from build123d import *

# Parameters (mm, degrees)
SKETCH_2_R      = 1.6
SKETCH_2_W      = 5
SKETCH_2_H      = 2
SKETCH_2_W_2    = 25.8
SKETCH_2_H_2    = 5
EXTRUDE_1_DEPTH = 1.6
SKETCH_3_W      = 5
SKETCH_3_H      = 25
SKETCH_3_W_2    = 7.5
SKETCH_3_H_2    = 5
SKETCH_3_W_3    = 8
SKETCH_3_H_3    = 4.5
SKETCH_3_W_4    = 25
SKETCH_3_H_4    = 24.5
EXTRUDE_2_DEPTH = 2
SKETCH_4_R      = 1.5
EXTRUDE_3_DEPTH = 5
SKETCH_5_W      = 5.2
SKETCH_5_H      = 3
SKETCH_5_W_2    = 4.3
SKETCH_5_H_2    = 4.3
SKETCH_5_W_3    = 3
SKETCH_5_H_3    = 5.2
EXTRUDE_4_DEPTH = 2


with BuildPart() as part:
    # 草图2 → 凸台-拉伸1 (new body)
    with BuildSketch(Plane(origin=(0, 0, 0), x_dir=(1, 0, 0), z_dir=(0, 1, 0))):
        Polygon((0, 0), (0, -53), (8, -53), (8, -37), (26, -37), (26, -53), (91, -53), (91, 0), align=None)
        with Locations(Location((3, -50, 0), (0, 0, 270))):
            Circle(SKETCH_2_R, mode=Mode.SUBTRACT)
        with Locations(Location((3, -3, 0), (0, 0, 270))):
            Circle(SKETCH_2_R, mode=Mode.SUBTRACT)
        with Locations(Location((88, -30, 0), (0, 0, 270))):
            Circle(SKETCH_2_R, mode=Mode.SUBTRACT)
        with Locations(Location((88, -50, 0), (0, 0, 270))):
            Circle(SKETCH_2_R, mode=Mode.SUBTRACT)
        with Locations((14, -33)):
            Rectangle(SKETCH_2_W, SKETCH_2_H, mode=Mode.SUBTRACT)
        with Locations((70.1, -38.9)):
            Rectangle(SKETCH_2_W_2, SKETCH_2_H_2, mode=Mode.SUBTRACT)
    extrude(amount=EXTRUDE_1_DEPTH)

    # 草图3 → 凸台-拉伸2 (add)
    with BuildSketch(Plane(origin=(0, 1.6, 0), x_dir=(1, 0, 0), z_dir=(0, 1, 0))):
        with Locations((2.5, -26.5)):
            Rectangle(SKETCH_3_W, SKETCH_3_H)
        with Locations((14.05, -18)):
            Rectangle(SKETCH_3_W_2, SKETCH_3_H_2)
        with Locations((22, -32.25)):
            Rectangle(SKETCH_3_W_3, SKETCH_3_H_3)
        with Locations((69.5, -18)):
            Rectangle(SKETCH_3_W_4, SKETCH_3_H_2)
        with Locations((88.5, -13.75)):
            Rectangle(SKETCH_3_W, SKETCH_3_H_4)
    extrude(amount=EXTRUDE_2_DEPTH)

    # 草图4 → 凸台-拉伸3 (add)
    with BuildSketch(Plane(origin=(0, 1.6, 0), x_dir=(1, 0, 0), z_dir=(0, 1, 0))):
        with Locations(Location((34.5, -38.8, 0), (0, 0, 270))):
            Circle(SKETCH_4_R)
        with Locations(Location((38.1, -38.8, 0), (0, 0, 270))):
            Circle(SKETCH_4_R)
        with Locations(Location((41.7, -38.8, 0), (0, 0, 270))):
            Circle(SKETCH_4_R)
    extrude(amount=EXTRUDE_3_DEPTH)

    # 草图5 → 凸台-拉伸4 (add)
    with BuildSketch(Plane(origin=(0, 1.6, 0), x_dir=(1, 0, 0), z_dir=(0, 1, 0))):
        with Locations((39.5, -43.5)):
            Rectangle(SKETCH_5_W, SKETCH_5_H)
        with Locations((49.05, -44.25)):
            Rectangle(SKETCH_5_W_2, SKETCH_5_H_2)
        with Locations((53.1, -40.8)):
            Rectangle(SKETCH_5_W_3, SKETCH_5_H_3)
    extrude(amount=EXTRUDE_4_DEPTH)


solid = part.part
Part model, mm, in its own coordinate system. A direction names the side the tool comes from. Coordinates: 2 decimals unless noted, no trailing zeros. Loops run counter-clockwise (first coordinate to the right, second up) from the corner with the lowest first, then second, coordinate; pieces in that order, holes last. Notation, with made-up numbers: M 16,75 L 75,75 A10 cw 75,91 Z; hole C 23.5,51.25 d4. An arc over 180 degrees is marked long. Use a Markdown table: item, result. Add a question column.
Q1. Pin check, flat tips, straight feed: P1, Ø10, axis at x = 81.5, z = 20, coming from the -Y side; P2, Ø1.5, axis at x = 52.5, z = 41, coming from the +Y side; P3, Ø1, axis at x = 60.5, y = 4, coming from the -Z side; P4, Ø0.8, axis at x = 14, y = 0.5, coming from the +Z side. Stop position of each tip, or through.
Q2. Cut at D-D (x = 38.1). Write the cut outline in (y, z), and give its area (3 significant figures).
Q3. Probe L1, parallel to X at y = 3, z = 17; L2, parallel to X at y = 1.1, z = 50; L3, parallel to Z at x = 62.5, y = 1.5. List the from-to ranges inside material, lowest first.
Q4. Which spindle directions (+Z, -Z, +X, -X, +Y, -Y) get a long thin tool onto all of the face, cutting with end or side? Do faces 1 (the flat face through (22, 3, 34.5)), 2 (the flat face through (5, 3, 27)), 3 (the flat face through (2, 3, 14)). Say none if no direction does.
Q5. Cut at C-C (y = 5.5). Write the cut outline in (x, z), and give its area (3 significant figures).
Q6. Mould opens along Z. For faces 4 (the flat face through (69, 3.6, 18)), 5 (the flat face through (49, 3, 42.1)), 6 (the cylindrical face through (88.481, 0.789, 51.526)) say: +Z half, -Z half, draft (parallel to the pull), parting line (faces both ways), or undercut.
Q7. Cut at B-B (z = 3). Write the cut outline in (x, y).
Q8. Cut at A-A (x = 69). Write the cut outline in (y, z).
Worked out:
| question | item | result |
|---|---|---|
| 1 | P1 | stops at y = 0 |
| 1 | P2 | stops at y = 3.6 |
| 1 | P3 | stops at z = 15.5 |
| 1 | P4 | stops at z = 37 |
| 2 | outline | M 0,0 L 1.6,0 L 1.6,37.3 L 6.6,37.3 L 6.6,40.3 L 1.6,40.3 L 1.6,42 L 3.6,42 L 3.6,45 L 1.6,45 L 1.6,53 L 0,53 Z |
| 2 | area | 106 mm2 |
| 3 | L1 | x = 0 to 5, 10.3 to 17.8, 57 to 82, 86 to 91 |
| 3 | L2 | x = 0 to 1.4, 4.6 to 8, 26 to 86.4, 89.6 to 91 |
| 3 | L3 | z = 0 to 36.4, 41.4 to 53 |
| 4 | face 1 | +Z, +X, +Y |
| 4 | face 2 | +Z, -Z, +Y |
| 4 | face 3 | -Z, -X, +Y |
| 5 | outline | C 34.5,38.8 d3; C 38.1,38.8 d3; C 41.7,38.8 d3 |
| 5 | area | 21.2 mm2 |
| 6 | face 4 | draft |
| 6 | face 5 | -Z half |
| 6 | face 6 | undercut |
| 7 | outline | M 0,0 L 1.4,0 L 1.4,1.6 L 0,1.6 Z; M 4.6,0 L 91,0 L 91,3.6 L 86,3.6 L 86,1.6 L 4.6,1.6 Z |
| 8 | outline | M 0,0 L 1.6,0 L 1.6,15.5 L 3.6,15.5 L 3.6,20.5 L 1.6,20.5 L 1.6,36.4 L 0,36.4 Z; M 0,41.4 L 1.6,41.4 L 1.6,53 L 0,53 Z |
